Geometry: final body of the model. Coordinates: model frame, mm. Give positions to 0.01 mm unless a question says otherwise; leave off trailing zeros. Write each loop counter-clockwise with the first axis right and the second up, starting at its lowest first coordinate (ties: lowest second). Pieces come first, ordered by that corner, then holes. Notation, with made-up numbers: (87.5, -39.75) -> (132.5, -39.75) arc R27 ccw to (132.5, -4.75) -> close; hole circle Ø2 at (16.5, 18). An arc over 180 degrees is marked (long way). Answer in a Markdown table with one row per item. Add a question column.
Item 1: First-contact query: P1, Ø1.3, axis at x = -1, z = -0.5, coming from the -Y side; P2, Ø0.6, axis at y = 1, z = -0.5, coming from the +X side; P3, Ø1, axis at x = 1, y = 2, coming from the +Z side; P4, Ø1.5, axis at x = -1.5, y = 1.5, coming from the -Z side. Flat tips, straight axial feed; report the tip coordinate or a pass-through.
Item 2: Section query B-B on z = -4.5. Output: boundary loops of the cut face in (x, y).
Item 3: Section query A-A on z = -1.25. Output: boundary loops of the cut face in (x, y), plus the area to 3 significant figures.
Item 4: Draft query along X for faces 1 (the flat face through (0, -0.9, -0.8)), 2 (the flat face through (0, 0, -6.7)), 3 (the cylindrical face through (-0.07, -1.5, -5)). Return one class per face: +X half, -X half, draft (parallel to the pull), parting line (faces both ways), or undercut.
Item 5: Material intervals for probe 1 along X at (y, z) = (-0.4, -1.25); probe 2 along X at (y, z) = (-0.45, -3.5); probe 3 along Z at (x, y) = (-0.05, -0.15), sorted ascending. Write a range as from..to.
Autodesk Inventor part; units mm, degrees
ref_plane "WorkPlane2" through (0, 0, 0) normal (0, 0, 1) x (1, 0, 0)
ref_plane "Work Plane2" through (0, 0, -2.35) normal (0, 0, 1) x (1, 0, 0)
ref_plane "WorkPlane3" through (0, 0, 7) normal (0, 0, 1) x (1, 0, 0)
ref_plane "WorkPlane2" through (0, 0, 0) normal (0, 0, 1) x (1, 0, 0)
sketch "Sketch1" plane through (0, 0, 0) normal (1, 0, 0) x (0, 1, 0)
  point P0 (0, 0)
ref_plane "Work Plane2" through (0, 0, -2.35) normal (0, 0, 1) x (1, 0, 0)
ref_plane "WorkPlane3" through (0, 0, 7) normal (0, 0, 1) x (1, 0, 0)
sketch "Sketch2" plane through (0, 0, 0) normal (0, 1, 0) x (-1, 0, 0)
  point P0 (0, 0)
sketch "Sketch3" plane through (0, 0, 0) normal (1, 0, 0) x (0, 1, 0)
  line L0 (1.5, -3.35) -> (1.25, -2.85)
  line L1 (1.5, -6.7) -> (1.5, -3.35)
  line L2 (0, -6.7) -> (1.5, -6.7)
  line L3 (0, 0) -> (0, -6.7)
  arc A0 (2.75, -0.7) -> (0, 0) centre (0, -5.7518) ccw
  line L4 (2.75, -0.85) -> (2.75, -0.7)
  line L5 (1.25, -2.35) -> (2.75, -0.85)
  line L6 (1.25, -2.85) -> (1.25, -2.35)
  line L7 (0, -31.6445) -> (0, 31.6445) construction
  line L8 (0, -31.6445) -> (0, 31.6445)
  line L9 (0, -44.3023) -> (0, 44.3023)
  dimension "d2" = 1.5
  dimension "d4" = 1.25
  dimension "d6" = 0.5
  dimension "d8" = 1.65
  dimension "d10" = 135
  dimension "d12" = 2.75
  dimension "d14" = 0
  dimension "d16" = 0.7
  dimension "d18" = 6
  dimension "d22" = 3.35
revolve "Revolution1" add sketch "Sketch3" angle 360 about axis through (0, 0, -31.6445) along (0, 0, 1)
fillet "Fillet1" radius 0.8 1 edges at (0, -1.25, -2.35)
sketch "Sketch4" plane through (0, 0, 0) normal (0, 1, 0) x (-1, 0, 0)
  line L0 (0, 0) -> (-1.7, 0)
  line L1 (0, -1.4167) -> (0, 0)
  line L2 (-1.7, 0) -> (-0.2833, -1.4167)
  line L3 (0, -6.9021) -> (0, 1.1504)
  arc A0 (2.75, -0.7) -> (-2.75, -0.7) centre (0, -5.7518) ccw
  line L4 (0, -1.4167) -> (-0.2833, -1.4167)
  point P0 (0, -1.7)
  dimension "d30" = 45
  dimension "d33" = 3.4
  dimension "d34" = 0.2833
  dimension "d35" = 90
extrude "Extrusion1" cut sketch "Sketch4" along normal mid plane 0.5667
pattern_circular "PolarArray1" count 4 over 360 about axis through (0, 0, -10) along (0, 0, 1) of "Extrusion1"
thread "Thread1"
ref_plane "MSC_PF1" through (0, 0, 0) normal (1, 0, 0) x (0, 1, 0)
ref_plane "MSC_PT1" through (0, 2.75, -0.85) normal (0, 0, -1) x (-1, 0, 0)
equation "\"d2\" = 0.5 * NND"
equation "\"d4\" = 0.5 * msp_mdtds"
equation "\"d6\" = msp_x"
equation "\"d8\" = ParK"
equation "\"d12\" = 0.5 * Dk"
equation "\"d16\" = ParF"
equation "\"d18\" = NLG"
equation "\"d22\" = b"
equation "\"d24\" = r"
equation "\"d33\" = M"
equation "\"d31\" = 0.166667 * M"
equation "\"d39\" = b"
equation "\"PTC\" = 0.5"
equation "\"msp_x\" = PTC"
equation "\"NLG\" = 6"
equation "\"NND\" = 3"
equation "\"ParK\" = 1.65"
equation "\"r\" = 0.8"
equation "\"msp_mdtds\" = NND - PTC"
equation "\"b\" = 3.35"
equation "\"Dk\" = 5.5"
equation "\"ParF\" = 0.7"
equation "\"M\" = 3.4"
equation "\"ParA\" = 1"
equation "\"THREADDIA\" = NND"
equation "\"TEMPLATE\" = 1.2345"
properties part number "ISO 7047 - M3x6 - 4.8 - H" material "Steel"
Findings below:
| question | item | result |
|---|---|---|
| 1 | P1 | stops at y = -2.72 |
| 1 | P2 | stops at x = 2.64 |
| 1 | P3 | stops at z = -0.27 |
| 1 | P4 | stops at z = -6.7 |
| 2 | outline | circle Ø3 at (0, 0) |
| 3 | outline | circle Ø4.7 at (0, 0); hole (-0.45, -0.28) -> (-0.28, -0.28) -> (-0.28, -0.45) -> (0.28, -0.45) -> (0.28, -0.28) -> (0.45, -0.28) -> (0.45, 0.28) -> (0.28, 0.28) -> (0.28, 0.45) -> (-0.28, 0.45) -> (-0.28, 0.28) -> (-0.45, 0.28) -> close |
| 3 | area | 16.7 mm^2 |
| 4 | face 1 | undercut |
| 4 | face 2 | draft |
| 4 | face 3 | parting line |
| 5 | probe 1 | x = -2.32..-0.28, 0.28..2.32 |
| 5 | probe 2 | x = -1.43..1.43 |
| 5 | probe 3 | z = -6.7..-1.42 |
